```python
from build123d import *

# Parameters (mm, degrees)
SKETCH1_R           = 8.466666667
BOSS_EXTRUDE1_DEPTH = 3.96875
SCALE1_SCALE        = 0.75


with BuildPart() as part:
    # Sketch1 → Boss-Extrude1 (new body)
    with BuildSketch(Plane.XY):
        with BuildLine():
            Line((-12.7, 0), (-12.7, 127))
            ThreePointArc((-12.7, 127), (0, 139.7), (12.7, 127))
            Line((12.7, 127), (12.7, 0))
            ThreePointArc((12.7, 0), (0, -12.7), (-12.7, 0))
        make_face()
        Circle(SKETCH1_R, mode=Mode.SUBTRACT)
        with Locations((0, 127)):
            Circle(SKETCH1_R, mode=Mode.SUBTRACT)
    extrude(amount=BOSS_EXTRUDE1_DEPTH)


with BuildPart() as part_1:
    # Scale1: scaled about (0, 63.5, 1.984375)
    add(part.part.scale(SCALE1_SCALE).moved(Location((0, 15.875, 0.49609375))))


solid = part_1.part
```
Geometry check sheet. Reference: the model listing, model coordinates, mm. Give positions to 0.01 mm unless a question says otherwise; leave off trailing zeros. Loops run counter-clockwise (first coordinate to the right, second up) from the corner with the lowest first, then second, coordinate; pieces in that order, holes last. Notation, with made-up numbers: (70, 2.5) - (122, 2.5) arc R15 ccw to (122, 7.5) - close; hole circle Ø11 at (-3.5, 78). An arc over 180 degrees is marked (long way). Use CSV: the item, a comma, the result in double quotes. Start each with the question number.
Q1. Go/stop test with a flat-tipped pin: pin 1 Ø10 at (x, y) = (0, 111.125) entering from +Z. Record where the tip stops, or that it passes through.
Q2. Section check A-A, the plane x = 0. Record the cut outline in (y, z) (3 decimals), and give its area (3 significant figures).
Q3. Section check D-D, the plane x = 8. Record the cut outline in (y, z), and give its area (3 significant figures).
Q4. Section check C-C, the plane z = 1. Record the cut outline in (x, y) (3 decimals).
Q5. Section check B-B, the plane y = 113.5. Record the cut outline in (x, z).
Q6. Scan lines: probe 1 along Y at (x, z) = (0, 2.2) (3 decimals); probe 2 along Y at (x, z) = (-2, 1.3); probe 3 along X at (y, z) = (16.5, 0.7) (3 decimals). Record each from-to range of solid material in increasing order. Write a range as from..to.
Q7. Release check for a two-part mould opening along X. For faces 1 (the face through (0, 64, 0.496)), 2 (the face through (-1.377, 104.926, 1.964)), 3 (the face through (-0.209, 120.648, 1.964)) record: +X half, -X half, draft (parallel to the pull), parting line (faces both ways), or undercut.
Findings below:
1,pin 1,"passes through"
2,outline,"(6.35, 0.496) - (9.525, 0.496) - (9.525, 3.473) - (6.35, 3.473) - close; (22.225, 0.496) - (104.775, 0.496) - (104.775, 3.473) - (22.225, 3.473) - close; (117.475, 0.496) - (120.65, 0.496) - (120.65, 3.473) - (117.475, 3.473) - close"
2,area,"265 mm^2"
3,outline,"(10.71, 0.5) - (116.29, 0.5) - (116.29, 3.47) - (10.71, 3.47) - close"
3,area,"314 mm^2"
4,outline,"(-9.525, 15.875) arc R9.525 ccw to (9.525, 15.875) - (9.525, 111.125) arc R9.525 ccw to (-9.525, 111.125) - close; hole circle Ø12.7 at (0, 15.875); hole circle Ø12.7 at (0, 111.125)"
5,outline,"(-9.22, 0.5) - (-5.89, 0.5) - (-5.89, 3.47) - (-9.22, 3.47) - close; (5.89, 0.5) - (9.22, 0.5) - (9.22, 3.47) - (5.89, 3.47) - close"
6,probe 1,"y = 6.35..9.525, 22.225..104.775, 117.475..120.65"
6,probe 2,"y = 6.56..9.85, 21.9..105.1, 117.15..120.44"
6,probe 3,"x = -9.525..-6.319, 6.319..9.525"
7,face 1,"draft"
7,face 2,"undercut"
7,face 3,"parting line"
